Autodesk Inventor part; units mm, degrees
ref_plane "YZ Plane" through (0, 0, 0) normal (1, 0, 0) x (0, 1, 0)
ref_plane "XZ Plane" through (0, 0, 0) normal (0, 1, 0) x (-1, 0, 0)
ref_plane "XY Plane" through (0, 0, 0) normal (0, 0, 1) x (1, 0, 0)
sketch "Sketch1" plane through (0, 0, 0) normal (0, 0, 1) x (1, 0, 0)
  circle A0 centre (0, 0) radius 52.025
  line L0 (-2.05, 56.1236) -> (2.05, 56.1236)
  line L1 (2.05, 56.1236) -> (2.05, 48.6562)
  line L2 (2.05, 48.6562) -> (-2.05, 48.6562)
  line L3 (-2.05, 48.6562) -> (-2.05, 56.1236)
  line L4 (0, 0) -> (0, 78.5962)
  circle A1 centre (0, 0) radius 51.475
  line L5 (-54.0102, 15.3935) -> (-52.7433, 19.2928)
  line L6 (-52.7433, 19.2928) -> (-45.6413, 16.9853)
  line L7 (-45.6413, 16.9853) -> (-46.9083, 13.0859)
  line L8 (-46.9083, 13.0859) -> (-54.0102, 15.3935)
  line L9 (-31.3302, -46.6099) -> (-34.6471, -44.2)
  line L10 (-34.6471, -44.2) -> (-30.2579, -38.1587)
  line L11 (-30.2579, -38.1587) -> (-26.9409, -40.5687)
  line L12 (-26.9409, -40.5687) -> (-31.3302, -46.6099)
  line L13 (34.6471, -44.2) -> (31.3302, -46.6099)
  line L14 (31.3302, -46.6099) -> (26.9409, -40.5687)
  line L15 (26.9409, -40.5687) -> (30.2579, -38.1587)
  line L16 (30.2579, -38.1587) -> (34.6471, -44.2)
  line L17 (52.7433, 19.2928) -> (54.0102, 15.3935)
  line L18 (54.0102, 15.3935) -> (46.9083, 13.0859)
  line L19 (46.9083, 13.0859) -> (45.6413, 16.9853)
  line L20 (45.6413, 16.9853) -> (52.7433, 19.2928)
  point P0 (2.05, 51.4342)
  point P1 (-2.05, 51.4342)
  point P2 (-2.05, 51.9846)
  point P3 (-48.8068, 18.0138)
  point P4 (-48.2833, 17.8437)
  point P5 (-49.5503, 13.9444)
  point P6 (-50.0738, 14.1145)
  point P7 (-32.2143, -40.8515)
  point P8 (-31.8907, -40.4062)
  point P9 (-28.5738, -42.8161)
  point P10 (-28.8973, -43.2614)
  point P11 (28.8973, -43.2614)
  point P12 (28.5738, -42.8161)
  point P13 (31.8907, -40.4062)
  point P14 (32.2143, -40.8515)
  point P15 (50.0738, 14.1145)
  point P16 (49.5503, 13.9444)
  point P17 (48.2833, 17.8437)
  point P18 (48.8068, 18.0138)
  point P19 (2.05, 51.9846)
  dimension "d0" = 104.05
  dimension "d2" = 0.55
  dimension "d3" = 2.05
  dimension "d4" = 4.1
  dimension "d7" = 360
extrude "Extrusion1" add sketch "Sketch1" along normal blind 13 contours A0 L16 A1 L18 | L20 A1 L1 A0 | L18 L19 L20 A1 | A1 L16 L15 L14 L12 L11 L10 L8 L7 L6 L3 L2 L1 L20 L19 L18 | A0 L12 A1 L14 | A1 L14 L15 L16 | L1 L2 L4 A1 | A0 L8 A1 L10 | A1 L10 L11 L12 | L3 A1 L6 A0 | L4 L2 L3 A1 | A1 L6 L7 L8
chamfer "Chamfer1" distance 0.55 distance2 3.2 5 edges at (49.4787, -16.0766, 13) (0, -52.025, 13) (-49.4787, -16.0766, 13) (-30.5795, 42.0891, 13) (30.5795, 42.0891, 13) measured on face at (-10.4211, -2.2799, 13)
sketch "Sketch2" plane through (0, 0, 0) normal (0, 0, -1) x (-1, 0, 0)
  circle A0 centre (0, 0) radius 22
  dimension "d14" = 44
extrude "Extrusion2" add sketch "Sketch2" along normal blind 4
sketch "Sketch3" plane through (0, 0, 13) normal (0, 0, 1) x (1, 0, 0)
  circle A0 centre (0, 0) radius 34.95
  dimension "d17" = 69.9
extrude "Extrusion3" add sketch "Sketch3" along normal blind 9.9
sketch "Sketch4" plane through (0, 0, 22.9) normal (0, 0, 1) x (1, 0, 0)
  circle A0 centre (0, 0) radius 13.5
  dimension "d20" = 27
extrude "Extrusion4" add sketch "Sketch4" along normal blind 2.25
sketch "Sketch5" plane through (0, 0, 25.15) normal (0, 0, 1) x (1, 0, 0)
  circle A0 centre (0, 0) radius 7.5
  dimension "d23" = 15
extrude "Extrusion5" cut sketch "Sketch5" against normal through all
properties part number "main_motor_planet" material "Aluminum 6061-AHC"
Source: CAD feature listing. Evaluate the final solid. Frame: model axes, mm. A direction names the side the tool comes from. Round coordinates to 2 decimals unless told otherwise and drop trailing zeros. Write each loop counter-clockwise with the first axis right and the second up, starting at its lowest first coordinate (ties: lowest second). Pieces come first, ordered by that corner, then holes. Notation, with made-up numbers: (11, 26.5) - (42, 26.5) arc R22 cw to (42, 33.5) - close; hole circle Ø9 at (88.5, 81). An arc over 180 degrees is marked (long way). Use CSV: the item, a comma, the result in double quotes. Start each with the question number.
(1) Mould query, pull axis Y, two halves, no side actions, for faces 4 (the face through (0, -9, -4)), 5 (the face through (-49.344, -16.484, 4.832)), 6 (the face through (48.95, 15.93, 6.41)). Classes: pulls with the +Y half, pulls with the -Y half, needs draft (parallel to the pull), parting line crosses it, or undercut.
(2) Material intervals for probe 1 along Z at (x, y) = (-25.5, -7); probe 2 along X at (y, z) = (-1, 6.25); probe 3 along Z at (x, y) = (-10, -37.5), sorted ascending. Write a range as [from, to].
(3) Set-up query: faces 1 (the face through (0.43, -51.69, 11.73)), 2 (the face through (15, 0, 22.9)), 3 (the face through (22.4, 0.7, 0)). Return all of +Z, -Z, +X, -X, +Y, -Y with unobstructed straight access to the full face (end or side cutting, diameter ignored); none if empty.
(4) First-contact query: pin 1 Ø3 at (x, y) = (-38.5, -2.5) entering from +Z; pin 2 Ø4 at (y, z) = (-33, 0) entering from +X; pin 3 Ø10 at (x, y) = (-18.5, -24) entering from +Z. Flat tips, straight axial feed; report the tip coordinate or a pass-through.
(5) Cut plane C-C, the plane z = 19.5. Return loops of the section in (x, y).
Geometry says:
1,face 4,"needs draft"
1,face 5,"parting line crosses it"
1,face 6,"undercut"
2,probe 1,"[0, 22.9]"
2,probe 2,"[-52.02, -7.43], [7.43, 52.02]"
2,probe 3,"[0, 13]"
3,face 1,"+Z, -Y"
3,face 2,"+Z"
3,face 3,"-Z"
4,pin 1,"z = 13"
4,pin 2,"x = 41.78"
4,pin 3,"z = 22.9"
5,outline,"circle Ø69.9 at (0, 0); hole circle Ø15 at (0, 0)"
